Could you check a few things on this model? Use its own coordinates, in mm. Give positions to 0.01 mm unless a question says otherwise; leave off trailing zeros. Write each loop counter-clockwise with the first axis right and the second up, starting at its lowest first coordinate (ties: lowest second). Pieces come first, ordered by that corner, then holes. Notation, with made-up numbers: (-28, 50) - (-15, 50) arc R15 cw to (-15, 71) - close; hole circle Ø4 at (48, 12). An arc over 180 degrees is marked (long way). Answer as a JSON object with one key per item and string values. Group by question number.
Autodesk Inventor part; units mm, degrees
ref_plane "YZ Plane" through (0, 0, 0) normal (1, 0, 0) x (0, 1, 0)
ref_plane "XZ Plane" through (0, 0, 0) normal (0, 1, 0) x (-1, 0, 0)
ref_plane "XY Plane" through (0, 0, 0) normal (0, 0, 1) x (1, 0, 0)
sketch "Sketch2" plane through (0, 0, 0) normal (0, 0, 1) x (1, 0, 0)
  line L0 (-410.0497, 90.9112) -> (409.1003, 90.9112)
  line L1 (409.1003, 90.9112) -> (409.1003, -10.6888)
  line L2 (409.1003, -10.6888) -> (-410.0497, -10.6888)
  line L3 (-410.0497, -10.6888) -> (-410.0497, 90.9112)
  point P0 (0, 0)
  dimension "d0" = 819.15
  dimension "d1" = 101.6
extrude "Board" add sketch "Sketch2" along normal blind 19.05
sketch "Sketch10" plane through (0, 0, 19.05) normal (0, 0, 1) x (1, 0, 0)
  line L0 (409.1003, -10.6888) -> (409.1003, 90.9112)
  line L1 (409.1003, 81.3862) -> (-410.0497, 81.3862)
  line L2 (-410.0497, 81.3862) -> (-410.0497, 71.8612)
  line L3 (-410.0497, 71.8612) -> (409.1003, 71.8612)
  line L4 (409.1003, 71.8612) -> (409.1003, 81.3862)
  line L5 (-410.0497, 90.9112) -> (-410.0497, -10.6888)
  line L6 (409.1003, 90.9112) -> (-410.0497, 90.9112)
  point P0 (0, 0)
  dimension "d22" = 9.525
  dimension "d23" = 9.525
extrude "Extrusion7" cut sketch "Sketch10" against normal blind 9.525 contours L3 L2 L1 L0
sketch "Sketch11" plane through (-410.0497, 90.9112, 0) normal (0, 1, 0) x (1, 0, 0)
  line L0 (0, -19.05) -> (19.05, -19.05)
  line L1 (19.05, -19.05) -> (19.05, -9.525)
  line L2 (19.05, -9.525) -> (0, -9.525)
  line L3 (0, -9.525) -> (0, -19.05)
  line L4 (819.15, -9.525) -> (0, -9.525)
  line L5 (819.15, 0) -> (819.15, -19.05)
  line L6 (0, -9.525) -> (819.15, -9.525)
  line L7 (819.15, -19.05) -> (800.1, -19.05)
  line L8 (800.1, -19.05) -> (800.1, -9.525)
  line L9 (800.1, -9.525) -> (819.15, -9.525)
  line L10 (819.15, -9.525) -> (819.15, -19.05)
  point P0 (410.0497, 0)
  dimension "d28" = 19.05
  dimension "d29" = 19.05
extrude "End Notches" cut sketch "Sketch11" against normal blind 101.6
equation "\"d30\" = d1"
properties part number "Base Runner Front"
(1) I want a section at C-C, the plane x = 214. Please give me the cut outline in (y, z) (3 decimals).
(2) I want a section at A-A, the plane z = 13. Please give me the cut outline in (x, y).
(3) Will these pins go through, and if not, where does the flat tip stop? P1, Ø5, axis at y = 47.5, z = 16, coming from the +X side; P2, Ø7.5, axis at y = 48.5, z = 16, coming from the -X side.
(4) If we mould it in two halves opening along Y, with no side actions, what happens to faces 1 (the flat face through (1, 78, 9.525)), 2 (the flat face through (5, -10.689, 9)), 3 (the flat face through (-6, 90.911, 9)), 4 (the flat face through (-6, 31, 19.05))? For each: +Y half, -Y half, draft (parallel to the pull), parting line (faces both ways), or undercut.
(5) I want a section at B-B, the plane y = 50. Please give me the cut outline in (x, z) (3 decimals), and give its area (3 significant figures).
(6) I need wall thicknesses on L1, parallel to Y at x = -360.5, z = 17.25; L2, parallel to X at y = 25.5, z = 14.25; L3, parallel to Z at x = 349, y = 75 (3 decimals). Which ranges of each line are inside material? Lowest first, please.
Entries:
{
 "1": {"outline": "(-10.689, 0) - (90.911, 0) - (90.911, 19.05) - (81.386, 19.05) - (81.386, 9.525) - (71.861, 9.525) - (71.861, 19.05) - (-10.689, 19.05) - close"},
 "2": {"outline": "(-391, -10.69) - (390.05, -10.69) - (390.05, 71.86) - (-391, 71.86) - close; (-391, 81.39) - (390.05, 81.39) - (390.05, 90.91) - (-391, 90.91) - close"},
 "3": {"P1": "x = 390.05", "P2": "x = -391"},
 "4": {"face 1": "undercut", "face 2": "-Y half", "face 3": "+Y half", "face 4": "draft"},
 "5": {"outline": "(-410.05, 0) - (409.1, 0) - (409.1, 9.525) - (390.05, 9.525) - (390.05, 19.05) - (-391, 19.05) - (-391, 9.525) - (-410.05, 9.525) - close", "area": "15,200 mm^2"},
 "6": {"L1": "-10.69 to 71.86, 81.39 to 90.91", "L2": "-391 to 390.05", "L3": "0 to 9.525"}
}
